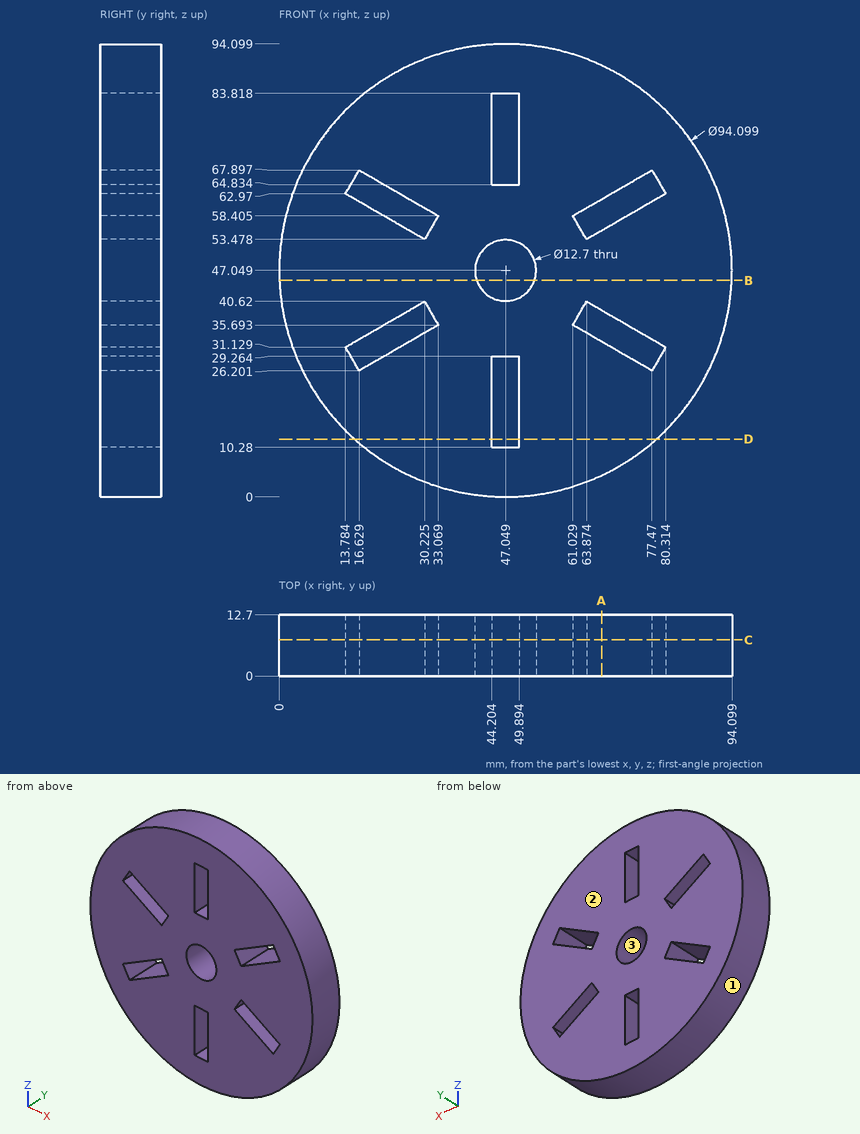
Geometry: see drawing. Coordinates: mm, zero at the bounding-box minimum. Round coordinates to 2 decimals unless told otherwise and drop trailing zeros. Order: outer loops, then holes, each group sorted by start corner. A loop starts at its lowest first (then second) coordinate and runs counter-clockwise, first axis right, second up. Notation, with made-up numbers: (1.5, 29.25) - (7.5, 29.25) arc R6 cw to (7.5, 33.25) - close; hole circle Ø4 at (-21.75, 31). An arc over 180 degrees is marked (long way). One line per question, with ' | ' between items. Start each with the question number.
1) Cut plane C-C, the plane y = 7.5. Give the number of separate pieces and of enclosed holes in the cut face, then the cut area to 3 significant figures.
2) Ray query, probe 1 along X at (y, z) = (6, 60) (1 decimal); probe 2 along X at (y, z) = (11.5, 36) (1 decimal); probe 3 along Z at (x, y) = (70.5, 6.25) (1 decimal). Return the intervals inside material, ascending.
3) Cut plane A-A, the plane x = 67. Return the cut outline in (y, z) (1 decimal).
4) Pull-direction query (Z, two-part tool) for the marked faces 1, 2 and 3; classes: +Z half, -Z half, draft (parallel to the pull), parting line (faces both ways), or undercut.
5) Cut plane D-D, the plane z = 12. Return the cut outline in (x, y) (1 decimal).
6) Cut plane B-B, the plane z = 45. Return the cut outline in (x, y) (1 decimal), then the cut area to 3 significant figures.
7) Contact query for flat-ended pins moving along their axis: P1, Ø1, axis at y = 3, z = 43, coming from the +X side (1 decimal); P2, Ø6.5, axis at x = 46.5, y = 8, coming from the +Z side; P3, Ø4.5, axis at x = 47, y = 3, coming from the -Z side; P4, Ø20.5, axis at x = 47.05, z = 47.05, coming from the +Y side. Output: stop coordinate, or through.
Worked out:
1) separate pieces: 1 | enclosed holes: 7 | area: 6,180 mm^2
2) probe 1: x = 1.8 to 18.9, 30.3 to 63.8, 75.2 to 92.3 | probe 2: x = 1.3 to 22.2, 32.9 to 61.2, 71.9 to 92.8 | probe 3: z = 6.3 to 30.2, 36.8 to 57.3, 63.9 to 87.8
3) outline: (0, 4.4) - (12.7, 4.4) - (12.7, 32.2) - (0, 32.2) - close; (0, 38.8) - (12.7, 38.8) - (12.7, 55.3) - (0, 55.3) - close; (0, 61.9) - (12.7, 61.9) - (12.7, 89.7) - (0, 89.7) - close
4) face 1: parting line | face 2: draft | face 3: undercut
5) outline: (15.7, 0) - (44.2, 0) - (44.2, 12.7) - (15.7, 12.7) - close; (49.9, 0) - (78.4, 0) - (78.4, 12.7) - (49.9, 12.7) - close
6) outline: (0, 0) - (41, 0) - (41, 12.7) - (0, 12.7) - close; (53.1, 0) - (94.1, 0) - (94.1, 12.7) - (53.1, 12.7) - close | area: 1,040 mm^2
7) P1: stops at x = 94 | P2: stops at z = 94.1 | P3: stops at z = 0 | P4: stops at y = 12.7
